Geometry check sheet. Reference: the model listing, model coordinates, mm. A direction names the side the tool comes from. Round coordinates to 2 decimals unless told otherwise and drop trailing zeros. Order: outer loops, then holes, each group sorted by start corner. A loop starts at its lowest first (then second) coordinate and runs counter-clockwise, first axis right, second up. Notation, with made-up numbers: (49.25, 69.25) - (104.25, 69.25) arc R27 ccw to (104.25, 100.25) - close; hole circle Ø4 at (-15.5, 5.5). An arc over 180 degrees is marked (long way). Write each question's results on one line, items separated by ' | '.
```python
from build123d import *

# Parameters (mm, degrees)
CHAMFER1_SIZE = 0.127


with BuildPart() as part:
    # Sketch1 → Revolve1 (revolve)
    with BuildSketch(Plane.XY, mode=Mode.PRIVATE) as revolve1_sk:
        Polygon((6.3627, 0), (44.45, 0), (44.45, 4.7625), (38.1, 4.7625), (38.1, 46.0375), (44.45, 46.0375), (44.45, 50.8), (6.3627, 50.8), (6.3627, 46.0248), (6.35, 46.0248), (6.35, 4.7752), (6.3627, 4.7752), align=None)
    revolve(revolve1_sk.sketch.rotate(Axis((0, 50.8, 0), (0, -1, 0)), 180), axis=Axis((0, 50.8, 0), (0, -1, 0)))

    # Chamfer1
    # the kernel refuses this chamfer: 0.127 mm, written as the material it takes off along each edge
    with BuildSketch(Plane(origin=(0, 46.0375, 0), x_dir=(-1, 0, 0), z_dir=(0, 0, 1))) as chamfer1_piece_1:
        Polygon((44.45 - CHAMFER1_SIZE, 0), (44.45, -CHAMFER1_SIZE), (44.45, 0), align=None)
    revolve(axis=Axis((0, 46.0375, 0), (0, -1, 0)), mode=Mode.SUBTRACT)
    with BuildSketch(Plane(origin=(0, 4.7625, 0), x_dir=(-1, 0, 0), z_dir=(0, 0, 1))) as chamfer1_piece_2:
        Polygon((44.45, CHAMFER1_SIZE), (44.45 - CHAMFER1_SIZE, 0), (44.45, 0), align=None)
    revolve(axis=Axis((0, 4.7625, 0), (0, -1, 0)), mode=Mode.SUBTRACT)
    with BuildSketch(Plane(origin=(0, 0, 0), x_dir=(-1, 0, 0), z_dir=(0, 0, 1))) as chamfer1_piece_3:
        Polygon((6.3627 + CHAMFER1_SIZE, 0), (6.3627, -CHAMFER1_SIZE), (6.3627, 0), align=None)
    revolve(axis=Axis((0, 0, 0), (0, -1, 0)), mode=Mode.SUBTRACT)
    with BuildSketch(Plane(origin=(0, 0, 0), x_dir=(-1, 0, 0), z_dir=(0, 0, 1))) as chamfer1_piece_4:
        Polygon((44.45 - CHAMFER1_SIZE, 0), (44.45, -CHAMFER1_SIZE), (44.45, 0), align=None)
    revolve(axis=Axis((0, 0, 0), (0, -1, 0)), mode=Mode.SUBTRACT)
    with BuildSketch(Plane(origin=(0, 46.0248, 0), x_dir=(-1, 0, 0), z_dir=(0, 0, 1))) as chamfer1_piece_5_section:
        Polygon((6.35 + CHAMFER1_SIZE, 0), (6.35, CHAMFER1_SIZE), (6.35, 0), align=None)
    chamfer1_piece_5 = revolve(axis=Axis((0, 46.0248, 0), (0, -1, 0)), mode=Mode.PRIVATE)
    chamfer1_piece_5 = chamfer1_piece_5 & Plane(origin=(0, 45.905383225, 0), x_dir=(-1, 0, 0), z_dir=(0, -1, 0)) * Cylinder(6.3627, 26, mode=Mode.PRIVATE)
    add(chamfer1_piece_5, mode=Mode.SUBTRACT)
    with BuildSketch(Plane(origin=(0, 4.7752, 0), x_dir=(-1, 0, 0), z_dir=(0, 0, 1))) as chamfer1_piece_6_section:
        Polygon((6.35, -CHAMFER1_SIZE), (6.35 + CHAMFER1_SIZE, 0), (6.35, 0), align=None)
    chamfer1_piece_6 = revolve(axis=Axis((0, 4.7752, 0), (0, -1, 0)), mode=Mode.PRIVATE)
    chamfer1_piece_6 = chamfer1_piece_6 & Plane(origin=(0, 4.894616775, 0), x_dir=(-1, 0, 0), z_dir=(0, -1, 0)) * Cylinder(6.3627, 26, mode=Mode.PRIVATE)
    add(chamfer1_piece_6, mode=Mode.SUBTRACT)
    with BuildSketch(Plane(origin=(0, 50.8, 0), x_dir=(-1, 0, 0), z_dir=(0, 0, 1))) as chamfer1_piece_7:
        Polygon((44.45, CHAMFER1_SIZE), (44.45 - CHAMFER1_SIZE, 0), (44.45, 0), align=None)
    revolve(axis=Axis((0, 50.8, 0), (0, -1, 0)), mode=Mode.SUBTRACT)
    with BuildSketch(Plane(origin=(0, 50.8, 0), x_dir=(-1, 0, 0), z_dir=(0, 0, 1))) as chamfer1_piece_8:
        Polygon((6.3627 + CHAMFER1_SIZE, 0), (6.3627, CHAMFER1_SIZE), (6.3627, 0), align=None)
    revolve(axis=Axis((0, 50.8, 0), (0, -1, 0)), mode=Mode.SUBTRACT)


solid = part.part
```
(1) Access from +Z, -Z, +X, -X, +Y, -Y to the whole of each face (thin tool, end or side, straight path). Record for faces 1 (the face through (19.5, 46.038, -33)), 2 (the face through (0.83, 48.26, -6.31)).
Answers follow:
face 1: none | face 2: +Y, -Y
(2) Material ranges on line 1 (Y direction, x = -37.5, z = 14); line 2 (Z direction, x = 0, y = 26); line 3 (Z direction, x = 0, y = 2.45), recorded low to high.
Answers follow:
line 1: 0 to 4.76, 46.04 to 50.8 | line 2: -38.1 to -6.35, 6.35 to 38.1 | line 3: -44.45 to -6.36, 6.36 to 44.45
(3) Draft check along Z on faces 3 (the face through (32.8, 48.5, -30)), 4 (the face through (-1, 0, 9)), 5 (the face through (-2.93, 25.113, 5.634)). Enter one of: released by +Z, released by -Z, zero draft, split by the parting line, or undercut.
Answers follow:
face 3: split by the parting line | face 4: zero draft | face 5: undercut
(4) Section check B-B (y = 48). Record the cut outline in (x, z).
Answers follow:
outline: circle Ø88.9 at (0, 0); hole circle Ø12.73 at (0, 0)
(5) Section check A-A (y = 21.5). Record the cut outline in (x, z).
Answers follow:
outline: circle Ø76.2 at (0, 0); hole circle Ø12.7 at (0, 0)
(6) Depth check by flat-ended pin: pin 1 Ø6 at (x, y) = (-31, 16.5) entering from -Z; pin 2 Ø11.5 at (x, z) = (0, 0) entering from -Y; pin 3 Ø4 at (y, z) = (15, 20.5) entering from -X; pin 4 Ø2 at (x, y) = (-33, 30) entering from +Z. Enter the tip coordinate at first touch or a pass-through.
Answers follow:
pin 1: z = -25.84 | pin 2: through | pin 3: x = -33.31 | pin 4: z = 20.68
